Geometry check sheet. Reference: the model listing, model coordinates, mm. Face numbers are marked on the shaded views. A direction names the side the tool comes from. Round coordinates to 2 decimals unless told otherwise and drop trailing zeros. Answer in a Markdown table with one row per item. Add a question column.
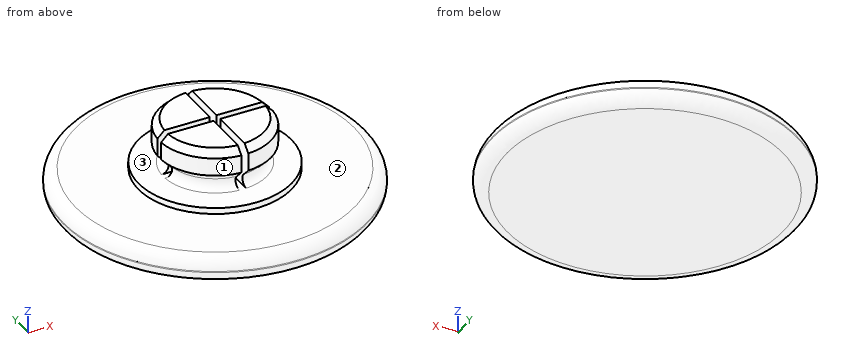
```python
from build123d import *

# Parameters (mm, degrees)
F2_R     = 0.5
F3_R     = 0.9
F4_SIZE  = 0.5
F6_DEPTH = 3.3


with BuildPart() as f1:
    # F0 (on Front) → F1 (revolve)
    with BuildSketch(Plane.XZ):
        with BuildLine():
            ThreePointArc((0, 0.7), (5.511125, 0.524823), (11, 0))
            Line((11, 0), (11, 2))
            Line((11, 2), (5.55, 2))
            Line((5.55, 2), (5.55, 2.45))
            Line((5.55, 2.45), (2.55, 2.45))
            Line((2.55, 2.45), (4.05, 3.95))
            Line((4.05, 3.95), (4.05, 5.75))
            Line((4.05, 5.75), (0, 5.75))
            Line((0, 5.75), (0, 0.7))
        make_face()
    revolve(axis=Axis((0, 0, 3.225), (0, 0, -1)))

    # F2
    f2_edges = [f1.edges().sort_by_distance(p)[0] for p in [
        (-2.55, 0, 2.45),
    ]]
    fillet(f2_edges, radius=F2_R)

    # F3
    f3_edges = [f1.edges().sort_by_distance(p)[0] for p in [
        (-11, 0, 0),
        (-11, 0, 2),
    ]]
    fillet(f3_edges, radius=F3_R)

    # F4
    f4_edges = [f1.edges().sort_by_distance(p)[0] for p in [
        (-4.05, 0, 5.75),
    ]]
    chamfer(f4_edges, length=F4_SIZE)

    # F5 (on face) → F6 (cut, through all)
    with BuildSketch(Plane.XY.offset(5.75)):
        Polygon((0.25, 4.5), (-0.25, 4.5), (-0.25, 0.25), (-4.5, 0.25), (-4.5, -0.25), (-0.25, -0.25), (-0.25, -4.5), (0.25, -4.5), (0.25, -0.25), (4.5, -0.25), (4.5, 0.25), (0.25, 0.25), align=None)
    extrude(amount=-F6_DEPTH, mode=Mode.SUBTRACT)


solid = f1.part
```
Q1. Depth check by flat-ended pin: P1, Ø1.7, axis at y = -1.5, z = 3.5, coming from the -X side; P2, Ø1, axis at x = 1, z = 3.5, coming from the -Y side; P3, Ø1.5, axis at x = 5, y = 7, coming from the -Z side. Enter the tip coordinate at first touch or a pass-through.
Q2. Set-up check for the marked faces 1, 2 and 3: record each of +Z, -Z, +X, -X, +Y, -Y from which the full face is reachable in a straight line by a thin tool's end or side.
Q3. Scan lines: line 1 (X direction, y = -2.5, z = 3.15); line 2 (Z direction, x = -5.25, y = -8.75); line 3 (Y direction, x = 0, z = 2.4). Record each from-to range of solid material in increasing order. Write a range as from..to.
Check sheet entries:
| question | item | result |
|---|---|---|
| 1 | P1 | x = -3.97 |
| 1 | P2 | y = -3.97 |
| 1 | P3 | z = 0.19 |
| 2 | face 1 | +Z, -X, -Y |
| 2 | face 2 | +Z |
| 2 | face 3 | none |
| 3 | line 1 | -2.15..-0.25, 0.25..2.15 |
| 3 | line 2 | 0.12..1.99 |
| 3 | line 3 | -5.55..5.55 |
